Here's how the part is built. I have some questions about the finished solid (model axes, mm). A direction names the side the tool comes from. Round coordinates to 2 decimals unless told otherwise and drop trailing zeros. Order: outer loops, then holes, each group sorted by start corner. A loop starts at its lowest first (then second) coordinate and runs counter-clockwise, first axis right, second up. Notation, with made-up numbers: (58, 60) -> (101, 60) arc R29 cw to (101, 99) -> close; hole circle Ø7 at (68.5, 87.25). An arc over 180 degrees is marked (long way). Use a Markdown table: item, result. Add a question column.
(1) I want a section at A-A, the plane x = 0. Please give me the cut outline in (y, z), then the cut area to 3 significant figures.
(2) Thinking about a two-plate mould opening in X: for faces 1 (the face through (0, 11.43, -18)), 2 (the face through (-18, 12.7, 0)), 3 (the face through (50.8, 6, 0)), which applies, pulls with the +X half, pulls with the -X half, needs draft (parallel to the pull), parting line crosses it, or undercut?
(3) I want a section at C-C, the plane y = 10. Please give me the cut outline in (x, z), then the cut area to 3 significant figures.
(4) If I drill on probe 1 along Z at (x, y) = (0, 9.5); probe 2 along X at (y, z) = (11.5, 13.5); probe 3 along Z at (x, y) = (11, 3), over which ranges is the centre line in solid material (lowest first)?
(5) I want a section at B-B, the plane z = 0. Please give me the cut outline in (x, y), then the cut area to 3 significant figures.
(6) On a 3-axis mill with a long thin cutter (end or side, diameter ignored), from which of +Z, -Z, +X, -X, +Y, -Y can I reach the whole of each face in a straight line? I mean faces 4 (the face through (33.24, 10.12, 0.36)), 5 (the face through (0, 11.43, 18)), 6 (the face through (8, 0, 12)), 7 (the face through (-37, 12.7, 0)), 8 (the face through (44.36, 2.57, -2.9)). Say none if no direction works.
(7) I'm going to push flat-ended pins straight in: P1, Ø6, axis at y = 5.5, z = -8, coming from the +X side; P2, Ø4, axis at x = 0.5, z = -17.5, coming from the +Y side. Where does each tip first touch, or does it pass through?
(8) I want a section at D-D, the plane y = 6.35. Please give me the cut outline in (x, z).
from build123d import *

# Parameters (mm, degrees)
F0_W     = 76.2
F0_H     = 50.8
F0_R     = 12.7
F1_DEPTH = 12.7
F2_W     = 6.35
F2_H     = 50.8
F3_DEPTH = 1.27
F5_DEPTH = 50.801
F6_R     = 4.7625
F7_DEPTH = 12.7


with BuildPart() as f1:
    # F0 (on Front) → F1 (new body)
    with BuildSketch(Plane.XZ):
        Rectangle(F0_W, F0_H)
        Circle(F0_R, mode=Mode.SUBTRACT)
    extrude(amount=-F1_DEPTH)

    # F2 (on face) → F3 (cut)
    with BuildSketch(Plane(origin=(0, 12.7, 0), x_dir=(-1, 0, 0), z_dir=(0, 1, 0))):
        with Locations((32.385, 0)):
            Rectangle(F2_W, F2_H)
        with BuildLine():
            Line((6.35, 10.9985226281), (6.35, 25.4))
            Line((6.35, 25.4), (-6.35, 25.4))
            Line((-6.35, 25.4), (-6.35, 10.9985226281))
            ThreePointArc((-6.35, 10.9985226281), (0, 12.7), (6.35, 10.9985226281))
        make_face()
        with BuildLine():
            Line((-6.35, -25.4), (6.35, -25.4))
            Line((6.35, -25.4), (6.35, -10.9985226281))
            ThreePointArc((6.35, -10.9985226281), (0, -12.7), (-6.35, -10.9985226281))
            Line((-6.35, -10.9985226281), (-6.35, -25.4))
        make_face()
    extrude(amount=-F3_DEPTH, mode=Mode.SUBTRACT)

    # F4 (on face) → F5 (cut, through all)
    with BuildSketch(Plane.XY.offset(25.4)):
        Polygon((31.75, 12.7), (19.05, 12.7), (16.1170606325, 7.62), (34.6829393675, 7.62), align=None)
    extrude(amount=-F5_DEPTH, mode=Mode.SUBTRACT)

    # F6 (on face) → F7 (join)
    with BuildSketch(Plane.YZ.offset(38.1)):
        with Locations((6.35, 0)):
            Circle(F6_R)
    extrude(amount=F7_DEPTH)


solid = f1.part
Taken from the geometry:
| question | item | result |
|---|---|---|
| 1 | outline | (0, -25.4) -> (11.43, -25.4) -> (11.43, -12.7) -> (0, -12.7) -> close; (0, 12.7) -> (11.43, 12.7) -> (11.43, 25.4) -> (0, 25.4) -> close |
| 1 | area | 290 mm2 |
| 2 | face 1 | undercut |
| 2 | face 2 | needs draft |
| 2 | face 3 | pulls with the +X half |
| 3 | outline | (-38.1, -25.4) -> (17.49, -25.4) -> (17.49, 25.4) -> (-38.1, 25.4) -> close; (33.31, -25.4) -> (38.1, -25.4) -> (38.1, -3.06) -> (50.8, -3.06) -> (50.8, 3.06) -> (38.1, 3.06) -> (38.1, 25.4) -> (33.31, 25.4) -> close; hole circle Ø25.4 at (0, 0) |
| 3 | area | 2,640 mm2 |
| 4 | probe 1 | z = -25.4 to -12.7, 12.7 to 25.4 |
| 4 | probe 2 | x = -38.1 to -35.56, -29.21 to -6.35, 6.35 to 18.36, 32.44 to 38.1 |
| 4 | probe 3 | z = -25.4 to -6.35, 6.35 to 25.4 |
| 5 | outline | (-38.1, 0) -> (-12.7, 0) -> (-12.7, 12.7) -> (-29.21, 12.7) -> (-29.21, 11.43) -> (-35.56, 11.43) -> (-35.56, 12.7) -> (-38.1, 12.7) -> close; (12.7, 0) -> (38.1, 0) -> (38.1, 1.59) -> (50.8, 1.59) -> (50.8, 11.11) -> (38.1, 11.11) -> (38.1, 12.7) -> (31.75, 12.7) -> (34.68, 7.62) -> (16.12, 7.62) -> (19.05, 12.7) -> (12.7, 12.7) -> close |
| 5 | area | 679 mm2 |
| 6 | face 4 | +Z, -Z |
| 6 | face 5 | +Z, -Z, +Y |
| 6 | face 6 | +Z, -Z, +X, -X, -Y |
| 6 | face 7 | +Z, -Z, +X, -X, +Y |
| 6 | face 8 | +X |
| 7 | P1 | stops at x = 38.1 |
| 7 | P2 | stops at y = 11.43 |
| 8 | outline | (-38.1, -25.4) -> (38.1, -25.4) -> (38.1, -4.76) -> (50.8, -4.76) -> (50.8, 4.76) -> (38.1, 4.76) -> (38.1, 25.4) -> (-38.1, 25.4) -> close; hole circle Ø25.4 at (0, 0) |
